Answer from the drawing. Dimensions are ordinates in mm from the lowest x, y and z of the part. Round coordinates to 2 decimals unless told otherwise and drop trailing zeros. Loops run counter-clockwise (first coordinate to the right, second up) from the corner with the lowest first, then second, coordinate; pieces in that order, holes last. Notation, with made-up numbers: (-34.5, 11.25) -> (5.5, 11.25) arc R18 cw to (5.5, 37.25) -> close; hole circle Ø2 at (-14.75, 27.5). An arc over 180 degrees is marked (long way). One line per question, with ' | ' between items.
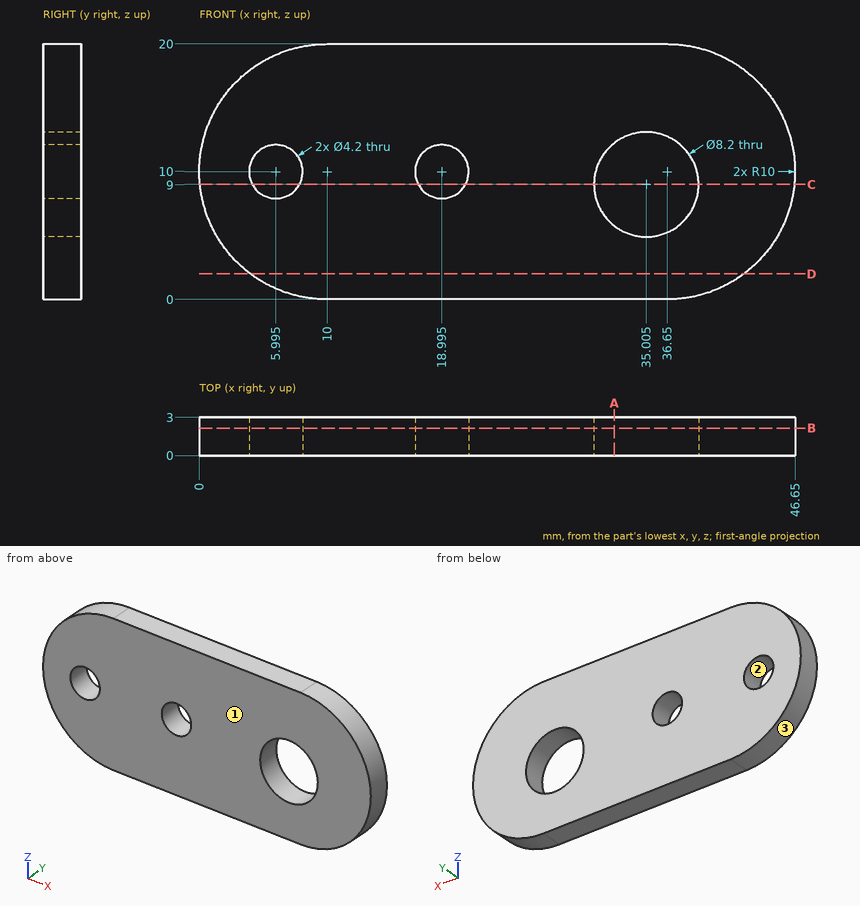
Q1. A cutting plane is placed at A-A on x = 32.5. Give the vertices of the cut face in (y, z).
Numbers:
outline: (0, 0) -> (3, 0) -> (3, 5.75) -> (0, 5.75) -> close; (0, 12.25) -> (3, 12.25) -> (3, 20) -> (0, 20) -> close
Q2. A cutting plane is placed at B-B on y = 2.15. Give the vertices of the cut face in (x, z) (3 decimals).
Numbers:
outline: (10, 0) -> (36.65, 0) arc R10 ccw to (36.65, 20) -> (10, 20) arc R10 ccw to start; hole circle Ø4.2 at (5.995, 10); hole circle Ø4.2 at (18.995, 10); hole circle Ø8.2 at (35.005, 9)
Q3. A cutting plane is placed at D-D on z = 2. Give the vertices of the cut face in (x, y), plus the area to 3 significant figures.
Numbers:
outline: (4, 0) -> (42.65, 0) -> (42.65, 3) -> (4, 3) -> close | area: 116 mm^2
Q4. Find the intervals of material crossed by line 1 (X direction, y = 1.85, z = 10) (3 decimals); line 2 (X direction, y = 2.25, z = 9) (3 decimals); line 3 (X direction, y = 0.3, z = 7.5), in increasing order. Write a range as from..to.
Numbers:
line 1: 0..3.895, 8.095..16.895, 21.095..31.029, 38.981..46.65 | line 2: 0.05..4.148, 7.842..17.148, 20.842..30.905, 39.105..46.6 | line 3: 0.32..31.19, 38.82..46.33
Q5. For a pull along X with two mould halves and no side action, classify the marked faces 1, 2 and 3 as pulls with the +X half, pulls with the -X half, needs draft (parallel to the pull), parting line crosses it, or undercut.
Numbers:
face 1: needs draft | face 2: undercut | face 3: pulls with the -X half
Q6. A cutting plane is placed at C-C on z = 9. Give the vertices of the cut face in (x, y) (3 decimals).
Numbers:
outline: (0.05, 0) -> (4.148, 0) -> (4.148, 3) -> (0.05, 3) -> close; (7.842, 0) -> (17.148, 0) -> (17.148, 3) -> (7.842, 3) -> close; (20.842, 0) -> (30.905, 0) -> (30.905, 3) -> (20.842, 3) -> close; (39.105, 0) -> (46.6, 0) -> (46.6, 3) -> (39.105, 3) -> close
